Study the drawing (mm; zero at the part's minimum x, y, z) and answer. A direction names the side the tool comes from. Give positions to 0.01 mm unless a question says otherwise; leave off trailing zeros. Write each loop counter-clockwise with the first axis right and the second up, starting at its lowest first coordinate (ties: lowest second). Pieces come first, ordered by that corner, then holes. Notation, with made-up numbers: (9.5, 58) -> (16.5, 58) arc R17 ccw to (16.5, 69) -> close; hole circle Ø3 at (78.5, 15). An arc over 180 degrees is marked (long way). One line per question, with ' | ' between items.
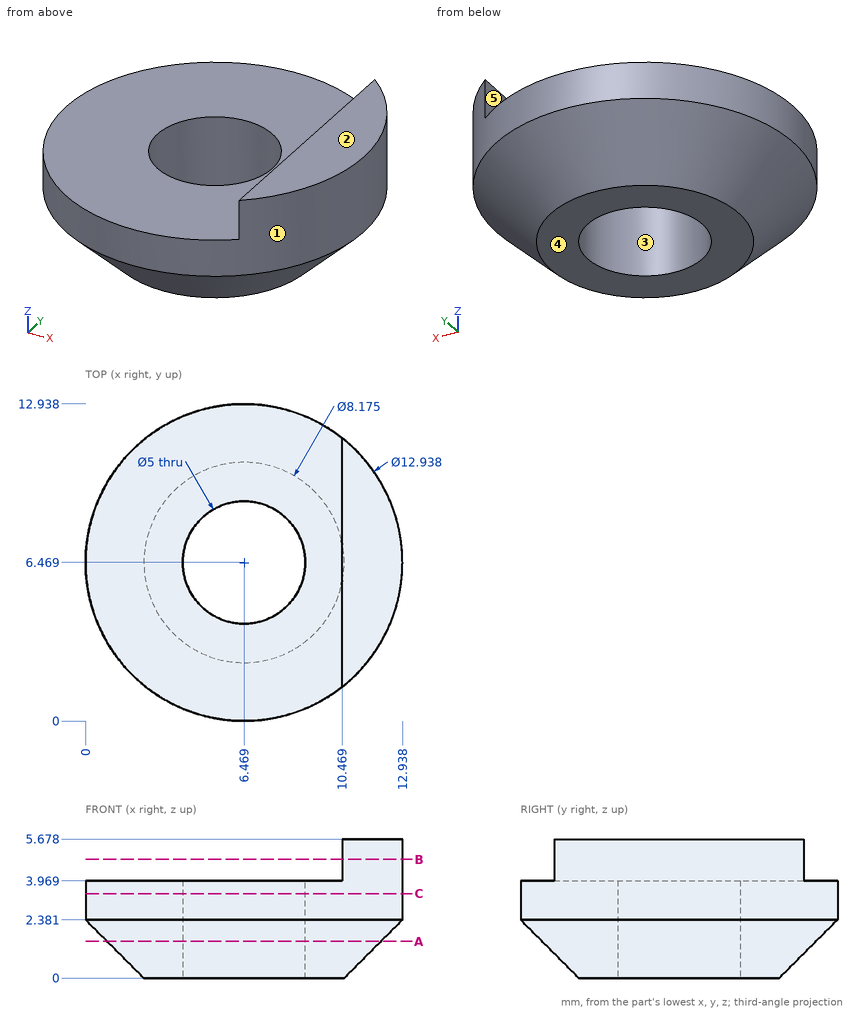
Item 1: Determine the mould class of the marked faces 1, 2 and 3 for opening direction Y: pulls with the +Y half, pulls with the -Y half, needs draft (parallel to the pull), parting line crosses it, or undercut.
Answers below:
face 1: parting line crosses it | face 2: needs draft | face 3: undercut
Item 2: Find section C-C (z = 3.45). Write down the section's boundary in (x, y), then the cut area to 3 significant figures.
Answers below:
outline: circle Ø12.94 at (6.47, 6.47); hole circle Ø5 at (6.47, 6.47) | area: 112 mm²
Item 3: Flat-ended cylindrical pins translate along their axes: pin 1 (6.5 mm diameter, centred on x = 6.47, y = 6.47, fed in from +Z); pin 2 (1 mm diameter, centred on y = 3.5, z = 2, fed in from +X); pin 3 (0.5 mm diameter, centred on y = 5.5, z = 4.5, fed in from -X). Find the tip coordinate at first contact, or state that the pin passes through.
Answers below:
pin 1: z = 3.97 | pin 2: x = 12.37 | pin 3: x = 10.47
Item 4: Find section A-A (z = 1.5). Write down the section's boundary in (x, y) (1 decimal).
Answers below:
outline: circle Ø11.2 at (6.5, 6.5); hole circle Ø5 at (6.5, 6.5)
Item 5: Find section B-B (z = 4.85). Write down the section's boundary in (x, y) (1 decimal), then the cut area to 3 significant figures.
Answers below:
outline: (10.5, 1.4) arc R6.5 ccw to (10.5, 11.6) -> close | area: 17.5 mm²
Item 6: A tool of negligible diameter and unlimited length cuts with its end or side. For the marked faces 4 and 5, from which of +Z, -Z, +X, -X, +Y, -Y can it reach the whole face along a straight path? Write none if from no direction.
Answers below:
face 4: -Z, +X, -X, +Y, -Y | face 5: +Z, -X, +Y, -Y
Item 7: Consider line 1 (Y direction, x = 7.25, z = 2.9) (1 decimal); line 2 (X direction, y = 7.25, z = 2) (1 decimal); line 3 (Y direction, x = 4.5, z = 3.85) (1 decimal). Determine where each line is inside the solid, lowest interval first. Write a range as [from, to].
Answers below:
line 1: [0, 4.1], [8.8, 12.9] | line 2: [0.4, 4.1], [8.8, 12.5] | line 3: [0.3, 4.9], [8, 12.6]
